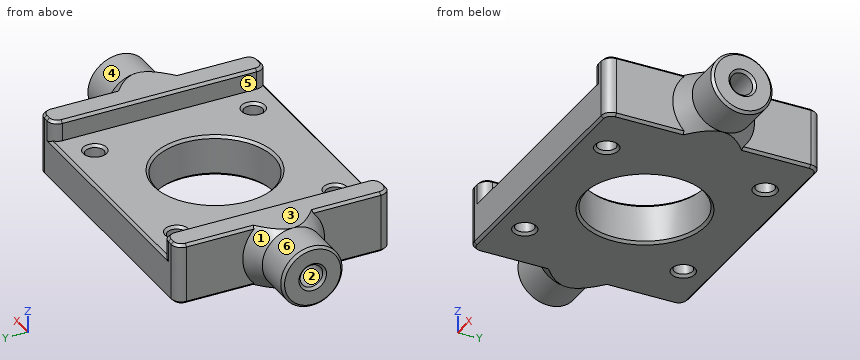
```python
from build123d import *

# Parameters (mm, degrees)
AUFSATZ_LINEAR_AUSTRAGEN1_DEPTH = 8
SKIZZE2_W                       = 5
SKIZZE2_H                       = 42
AUFSATZ_LINEAR_AUSTRAGEN2_DEPTH = 4
SKIZZE3_R                       = 6
AUFSATZ_LINEAR_AUSTRAGEN3_DEPTH = 11
SKIZZE5_R                       = 2.2
SCHNITT_LINEAR_AUSTRAGEN2_DEPTH = 10
SKIZZE4_R                       = 11.5
SKIZZE4_R_2                     = 1.8
SCHNITT_LINEAR_AUSTRAGEN1_DEPTH = 8
FASE1_SIZE                      = 2
FASE1_SIZE_2                    = 3.5
FASE2_SIZE                      = 2
FASE2_SIZE_2                    = 3.5
VERRUNDUNG1_R                   = 2
FASE3_SIZE                      = 0.5


with BuildPart() as part:
    # Skizze1 → Aufsatz-Linear austragen1 (new body)
    with BuildSketch(Plane.XY):
        Polygon((21, 21), (26, 21), (26, -21), (21, -21), (-21, -21), (-26, -21), (-26, 21), (-21, 21), align=None)
    extrude(amount=AUFSATZ_LINEAR_AUSTRAGEN1_DEPTH)

    # Skizze2 → Aufsatz-Linear austragen2 (add)
    with BuildSketch(Plane.XY.offset(8)):
        with Locations((23.5, 0)):
            Rectangle(SKIZZE2_W, SKIZZE2_H)
        with Locations((-23.5, 0)):
            Rectangle(SKIZZE2_W, SKIZZE2_H)
    extrude(amount=AUFSATZ_LINEAR_AUSTRAGEN2_DEPTH)

    # Skizze3 → Aufsatz-Linear austragen3 (add)
    with BuildSketch(Plane(origin=(26, 0, 0), x_dir=(0, 0, -1), z_dir=(1, 0, 0))):
        with Locations((-6, 0)):
            Circle(SKIZZE3_R)
    aufsatz_linear_austragen3 = extrude(amount=AUFSATZ_LINEAR_AUSTRAGEN3_DEPTH)

    # Skizze5 → Schnitt-Linear austragen2 (cut)
    with BuildSketch(Plane(origin=(37, 0, 0), x_dir=(0, 0, -1), z_dir=(1, 0, 0))):
        with Locations(Location((-6, 0, 0), (0, 0, 90))):
            Circle(SKIZZE5_R)
    schnitt_linear_austragen2 = extrude(amount=-SCHNITT_LINEAR_AUSTRAGEN2_DEPTH, mode=Mode.SUBTRACT)

    # Spiegeln1: Aufsatz-Linear austragen3, Schnitt-Linear austragen2 across plane
    add(aufsatz_linear_austragen3.mirror(Plane(origin=(0, 0, 0), x_dir=(0, 0, 1), z_dir=(1, 0, 0))))
    add(schnitt_linear_austragen2.mirror(Plane(origin=(0, 0, 0), x_dir=(0, 0, 1), z_dir=(1, 0, 0))), mode=Mode.SUBTRACT)

    # Skizze4 → Schnitt-Linear austragen1 (cut)
    with BuildSketch(Plane.XY.offset(8)):
        Circle(SKIZZE4_R)
        with Locations((-15.5, 15.5)):
            Circle(SKIZZE4_R_2)
        with Locations((15.5, 15.5)):
            Circle(SKIZZE4_R_2)
        with Locations((15.5, -15.5)):
            Circle(SKIZZE4_R_2)
        with Locations((-15.5, -15.5)):
            Circle(SKIZZE4_R_2)
    extrude(amount=-SCHNITT_LINEAR_AUSTRAGEN1_DEPTH, mode=Mode.SUBTRACT)

    # Fase1
    # the kernel refuses this chamfer: 3.5, 2 mm, written as the material it adds along each edge
    with BuildSketch(Plane(origin=(26, 0, 6), x_dir=(0, 0, -1), z_dir=(0, -1, 0))) as fase1_piece_1_section:
        Polygon((6 + FASE1_SIZE, 0), (6, FASE1_SIZE_2), (6, 0), align=None)
    fase1_piece_1 = revolve(axis=Axis((26, 0, 6), (1, 0, 0)), revolution_arc=180.000000388, mode=Mode.PRIVATE)
    fase1_piece_1 = split(fase1_piece_1, bisect_by=Plane(origin=(27.731298747, 6.967272798, 0), z_dir=(0, 0, 1)), keep=Keep.TOP, mode=Mode.PRIVATE)
    fase1_piece_1 = split(fase1_piece_1, bisect_by=Plane(origin=(27.731298747, 6.967272798, 12), z_dir=(0, 0, -1)), keep=Keep.TOP, mode=Mode.PRIVATE)
    add(fase1_piece_1)
    with BuildSketch(Plane(origin=(26, 0, 6), x_dir=(0, -6.764954696085317e-09, 1.0), z_dir=(0, 1.0, 6.764954696085317e-09))) as fase1_piece_2_section:
        Polygon((6 + FASE1_SIZE, 0), (6, FASE1_SIZE_2), (6, 0), align=None)
    fase1_piece_2 = revolve(axis=Axis((26, 0, 6), (1, 0, 0)), revolution_arc=179.999999612, mode=Mode.PRIVATE)
    fase1_piece_2 = split(fase1_piece_2, bisect_by=Plane(origin=(27.731298743, -6.9672728, 0), z_dir=(0, 0, 1)), keep=Keep.TOP, mode=Mode.PRIVATE)
    fase1_piece_2 = split(fase1_piece_2, bisect_by=Plane(origin=(27.731298743, -6.9672728, 12), z_dir=(0, 0, -1)), keep=Keep.TOP, mode=Mode.PRIVATE)
    add(fase1_piece_2)

    # Fase2
    # the kernel refuses this chamfer: 3.5, 2 mm, written as the material it adds along each edge
    with BuildSketch(Plane(origin=(-26, 0, 6), x_dir=(0, 0, -1), z_dir=(0, -1, 0))) as fase2_piece_1_section:
        Polygon((6 + FASE2_SIZE, 0), (6, -FASE2_SIZE_2), (6, 0), align=None)
    fase2_piece_1 = revolve(axis=Axis((-26, 0, 6), (1, 0, 0)), revolution_arc=180.000000388, mode=Mode.PRIVATE)
    fase2_piece_1 = split(fase2_piece_1, bisect_by=Plane(origin=(-27.731298747, 6.967272798, 0), z_dir=(0, 0, 1)), keep=Keep.TOP, mode=Mode.PRIVATE)
    fase2_piece_1 = split(fase2_piece_1, bisect_by=Plane(origin=(-27.731298747, 6.967272798, 12), z_dir=(0, 0, -1)), keep=Keep.TOP, mode=Mode.PRIVATE)
    add(fase2_piece_1)
    with BuildSketch(Plane(origin=(-26, 0, 6), x_dir=(0, -6.764954696085317e-09, 1.0), z_dir=(0, 1.0, 6.764954696085317e-09))) as fase2_piece_2_section:
        Polygon((6 + FASE2_SIZE, 0), (6, -FASE2_SIZE_2), (6, 0), align=None)
    fase2_piece_2 = revolve(axis=Axis((-26, 0, 6), (1, 0, 0)), revolution_arc=179.999999612, mode=Mode.PRIVATE)
    fase2_piece_2 = split(fase2_piece_2, bisect_by=Plane(origin=(-27.731298743, -6.9672728, 0), z_dir=(0, 0, 1)), keep=Keep.TOP, mode=Mode.PRIVATE)
    fase2_piece_2 = split(fase2_piece_2, bisect_by=Plane(origin=(-27.731298743, -6.9672728, 12), z_dir=(0, 0, -1)), keep=Keep.TOP, mode=Mode.PRIVATE)
    add(fase2_piece_2)

    # Verrundung1
    verrundung1_edges = [part.edges().sort_by_distance(p)[0] for p in [
        (26, 21, 6),
        (26, -21, 6),
        (-26, -21, 6),
        (-26, 21, 6),
        (21, -21, 10),
        (21, 21, 10),
        (-21, 21, 10),
        (-21, -21, 10),
    ]]
    fillet(verrundung1_edges, radius=VERRUNDUNG1_R)

    # Fase3
    fase3_edges = [part.edges().sort_by_distance(p)[0] for p in [
        (-26, -12.145751311, 0),
        (-26, 12.145751311, 12),
        (-21, 0, 12),
        (0, -21, 0),
        (23.5, -21, 12),
        (-23.5, -21, 12),
        (-23.5, 21, 12),
        (-26, -12.145751311, 12),
        (-25.414213562, 20.414213562, 12),
        (-25.414213562, -20.414213562, 12),
        (-21.585786438, 20.414213562, 12),
        (-21.585786438, -20.414213562, 12),
        (21, 0, 12),
        (26, 12.145751311, 12),
        (23.5, 21, 12),
        (25.414213562, 20.414213562, 12),
        (25.414213562, -20.414213562, 12),
        (21.585786438, 20.414213562, 12),
        (21.585786438, -20.414213562, 12),
        (0, 21, 0),
        (-26, 12.145751311, 0),
        (26, -12.145751311, 0),
        (25.414213562, 20.414213562, 0),
        (-25.414213562, 20.414213562, 0),
        (25.414213562, -20.414213562, 0),
        (-25.414213562, -20.414213562, 0),
        (0, 21, 8),
        (0, -21, 8),
        (37, 0, 12),
        (37, -2.2, 6),
        (-37, 0, 12),
        (-37, -2.2, 6),
        (-17.3, -15.5, 0),
        (-17.3, -15.5, 8),
        (13.7, -15.5, 0),
        (13.7, -15.5, 8),
        (13.7, 15.5, 0),
        (13.7, 15.5, 8),
        (-17.3, 15.5, 0),
        (-17.3, 15.5, 8),
        (-11.5, 0, 0),
        (-11.5, 0, 8),
        (26, -12.145751311, 12),
        (26, 12.145751311, 0),
    ]]
    chamfer(fase3_edges, length=FASE3_SIZE)


solid = part.part
```
Build history of the part. All positions in model axes, mm. Face numbers are marked on the shaded views. A direction names the side the tool comes from. Give positions to 0.01 mm unless a question says otherwise; leave off trailing zeros. Order: outer loops, then holes, each group sorted by start corner. A loop starts at its lowest first (then second) coordinate and runs counter-clockwise, first axis right, second up. Notation, with made-up numbers: M 66.25,57 L 117.25,57 A5 cw 117.25,61 Z; hole C -3.75,-1 d2. An arc over 180 degrees is marked long. Return JSON: item names as keys, results as strings.
Q1. 3-axis set-ups, long thin cutter, end or side, ignore diameter. For the marked faces 4, 5 and 6: which of +Z, -Z, +X, -X, +Y, -Y reach the whole face in a straight line?
Answer list:
{"face 4": "+X", "face 5": "+Z, +Y, -Y", "face 6": "-X"}
Q2. Two-plate mould, pull along Y, no slides. Class the marked faces 1, 2 and 3: pulls with the +Y half, pulls with the -Y half, needs draft (parallel to the pull), parting line crosses it, or undercut.
Answer list:
{"face 1": "pulls with the +Y half", "face 2": "undercut", "face 3": "needs draft"}
Q3. Band-saw the part on C-C (y = -15.5). Count the separate pieces of the cut face and the enclosed holes in it, then the cut area to 3 significant figures.
Answer list:
{"separate pieces": "3", "enclosed holes": "0", "area": "397 mm^2"}
Q4. Band-saw the part on A-A (x = -15.5). Give the cut face in (y, z), then the cut area to 3 significant figures.
Answer list:
{"outline": "M -21,0.5 L -20.5,0 L -17.8,0 L -17.3,0.5 L -17.3,7.5 L -17.8,8 L -20.5,8 L -21,7.5 Z; M -13.7,0.5 L -13.2,0 L 13.2,0 L 13.7,0.5 L 13.7,7.5 L 13.2,8 L -13.2,8 L -13.7,7.5 Z; M 17.3,0.5 L 17.8,0 L 20.5,0 L 21,0.5 L 21,7.5 L 20.5,8 L 17.8,8 L 17.3,7.5 Z", "area": "277 mm^2"}
Q5. Wall check: probe 1 along Z at (x, y) = (32.75, 0); probe 2 along X at (y, z) = (-17, 6.75); probe 3 along Y at (x, z) = (0, 2.25). Give the ranges that are in metal, low to high. Write a range as from..to.
Answer list:
{"probe 1": "z = 0..3.8, 8.2..12", "probe 2": "x = -26..-16.49, -14.51..14.51, 16.49..26", "probe 3": "y = -21..-11.5, 11.5..21"}
Q6. Flat gauge pins, fed straight in: pin 1 (4.5 mm diameter, centred on x = -15.5, y = -15.5, fed in from -Z); pin 2 (1.5 mm diameter, centred on x = 26.5, z = 5, fed in from +Y); pin 3 (5.5 mm diameter, centred on y = -14.5, z = 4.5, fed in from -X). Where does each tip first touch, or does it go through?
Answer list:
{"pin 1": "stops at z = 0.05", "pin 2": "stops at y = 19.97", "pin 3": "stops at x = -26"}
Q7. Band-saw the part on B-B (x = 0). Give the cut face in (y, z), then the cut area to 3 significant figures.
Answer list:
{"outline": "M -21,0.5 L -20.5,0 L -12,0 L -11.5,0.5 L -11.5,7.5 L -12,8 L -20.5,8 L -21,7.5 Z; M 11.5,0.5 L 12,0 L 20.5,0 L 21,0.5 L 21,7.5 L 20.5,8 L 12,8 L 11.5,7.5 Z", "area": "151 mm^2"}
